Can you work these out from the model? Positions are in its coordinate system, mm. A direction names the side the tool comes from. Round coordinates to 2 decimals unless told otherwise and drop trailing zeros. Loops run counter-clockwise (first coordinate to the right, second up) from the corner with the lowest first, then second, coordinate; pieces in that order, holes last.
(1) Thinking about a two-plate mould opening in Z: for faces 1 (the face through (-44, 4, 2.5)), 2 (the face through (7.27, 2.46, -7.92)), 3 (the face through (-59, 5, 1.7)), 4 (the face through (-61.225, 5, 2)), which applies, released by +Z, released by -Z, zero draft, split by the parting line, or undercut?
(2) I want a section at B-B on x = -23.5. Write out the boundary of the cut face in (y, z).
(3) Which directions (+Z, -Z, +X, -X, +Y, -Y) give clear straight access to the entire face, cutting with the end or side of a thin tool? Please do faces 5 (the face through (-57.604, 4.93, 1.092)), 6 (the face through (-56, 5, 0.5)), 7 (the face through (-61.225, 5, -1)), 8 (the face through (-40.225, 9, 0)), 9 (the face through (-51, 10, -1)).
(4) If I drill on line 1 along X through (y, z) = (3.95, 0); line 2 along Z through (x, y) = (-43, 3.75); line 3 along Z through (x, y) = (-16.5, 3.5), over which ranges is the centre line in solid material (lowest first)?
(5) I want a section at D-D on x = 0. Write out the boundary of the cut face in (y, z).
(6) I want a section at C-C on y = 6. Write out the boundary of the cut face in (x, z), plus the area to 3 significant figures.
(7) Will these pins go through, and if not, where does the flat tip stop? pin 1 Ø12 at (x, z) = (-4.5, 2.5) entering from +Y; pin 2 Ø3 at (x, y) = (-50.5, 5) entering from +Z; pin 3 Ø0.5 at (y, z) = (3.5, 0) entering from -X (3 decimals); pin 4 Ø4 at (y, z) = (5.5, -4) entering from -X (3 decimals).
(8) I want a section at A-A on x = -54. Write out the boundary of the cut face in (y, z).
from build123d import *

# Parameters (mm, degrees)
SKETCH_1_R               = 12
SKETCH_1_R_2             = 10.75
RING_DEPTH               = 5
SKETCH_2_W               = 50
SKETCH_2_H               = 5
STICK_DEPTH              = 5
SKETCH_3_W               = 21
SKETCH_3_H               = 5
KEY_DEPTH                = 10
FILLET_1_R               = 5
FILLET_5_R               = 3
CUT_EXTRUDE_1_DEPTH      = 63.839058045
CUT_EXTRUDE_1_DEPTH_BACK = 63.839058045
FILLET_7_R               = 0.5


with BuildPart() as part:
    # Эскиз1 → ring (new body)
    with BuildSketch(Plane(origin=(0, 0, 0), x_dir=(1, 0, 0), z_dir=(0, 1, 0))):
        with Locations(Location((0, 0, 0), (0, 0, 270))):
            Circle(SKETCH_1_R)
        with Locations(Location((0, 0, 0), (0, 0, 270))):
            Circle(SKETCH_1_R_2, mode=Mode.SUBTRACT)
    extrude(amount=RING_DEPTH)

    # Эскиз2 → stick (add)
    with BuildSketch(Plane(origin=(0, 0, 0), x_dir=(1, 0, 0), z_dir=(0, 1, 0))):
        with Locations((-36.22497216, 0)):
            Rectangle(SKETCH_2_W, SKETCH_2_H)
    extrude(amount=STICK_DEPTH)

    # Эскиз3 → key (add)
    with BuildSketch(Plane(origin=(0, 0, 0), x_dir=(1, 0, 0), z_dir=(0, 1, 0))):
        with Locations((-50.72497216, 0)):
            Rectangle(SKETCH_3_W, SKETCH_3_H)
    extrude(amount=KEY_DEPTH)

    # Скругление1
    fillet_1_edges = [part.edges().sort_by_distance(p)[0] for p in [
        (-11.736694594, 2.5, 2.5),
        (-11.736694594, 2.5, -2.5),
    ]]
    fillet(fillet_1_edges, radius=FILLET_1_R)

    # Скругление5
    fillet_5_edges = [part.edges().sort_by_distance(p)[0] for p in [
        (-40.22497216, 5, 0),
    ]]
    fillet(fillet_5_edges, radius=FILLET_5_R)

    # Эскиз4 → Вытянуть1 (cut, two sides: drawn at the far end of the back side and taken through both)
    with BuildSketch(Plane(origin=(0, 2.5, 0), x_dir=(1, 0, 0), z_dir=(0, 1, 0)).offset(-CUT_EXTRUDE_1_DEPTH_BACK)):
        Polygon((-61.22497216, 0.5), (-41.22497216, 0.5), (-41.22497216, -0.5), (-42.388207879, -0.5), (-42.82497216, -1.7), (-44.62497216, -1.7), (-45.061736441, -0.5), (-46.22497216, -0.5), (-47.388207879, -0.5), (-47.82497216, -1.7), (-49.62497216, -1.7), (-50.061736441, -0.5), (-51.22497216, -0.5), (-52.388207879, -0.5), (-52.82497216, -1.7), (-54.62497216, -1.7), (-55.061736441, -0.5), (-56.22497216, -0.5), (-57.388207879, -0.5), (-57.82497216, -1.7), (-59.62497216, -1.7), (-60.061736441, -0.5), (-61.22497216, -0.5), align=None)
    extrude(amount=CUT_EXTRUDE_1_DEPTH + CUT_EXTRUDE_1_DEPTH_BACK, mode=Mode.SUBTRACT)

    # Скругление7
    fillet_7_edges = [part.edges().sort_by_distance(p)[0] for p in [
        (-38.240559231, 0, 2.5),
        (12, 0, 0),
        (-38.240559231, 0, -2.5),
        (-12.613175603, 0, 3.255626562),
        (-12.613175603, 0, -3.255626562),
    ]]
    fillet(fillet_7_edges, radius=FILLET_7_R)


solid = part.part
Filled sheet:
1. face 1: released by +Z
1. face 2: undercut
1. face 3: undercut
1. face 4: zero draft
2. outline: (0, -2) arc R0.5 ccw to (0.5, -2.5) - (5, -2.5) - (5, 2.5) - (0.5, 2.5) arc R0.5 ccw to (0, 2) - close
3. face 5: +Y, -Y
3. face 6: -X, +Y, -Y
3. face 7: +Z, -Z, -X, +Y, -Y
3. face 8: +Z, -Z, +X, +Y
3. face 9: +Z, -Z, +X, -X, +Y
4. line 1: x = -41.22 to -10.75, 10.75 to 12
4. line 2: z = -2.5 to -0.5, 1.7 to 2.5
4. line 3: z = -2.5 to 2.5
5. outline: (0, -11.5) arc R0.5 ccw to (0.5, -12) - (5, -12) - (5, -10.75) - (0, -10.75) - close; (0, 10.75) - (5, 10.75) - (5, 12) - (0.5, 12) arc R0.5 ccw to (0, 11.5) - close
6. outline: (-61.22, -2.5) - (-39.46, -2.5) - (-39.46, 2.5) - (-61.22, 2.5) - (-61.22, 0.5) - (-60.06, 0.5) - (-59.62, 1.7) - (-57.82, 1.7) - (-57.39, 0.5) - (-55.06, 0.5) - (-54.62, 1.7) - (-52.82, 1.7) - (-52.39, 0.5) - (-50.06, 0.5) - (-49.62, 1.7) - (-47.82, 1.7) - (-47.39, 0.5) - (-45.06, 0.5) - (-44.62, 1.7) - (-42.82, 1.7) - (-42.39, 0.5) - (-41.22, 0.5) - (-41.22, -0.5) - (-61.22, -0.5) - close
6. area: 78.1 mm2
7. pin 1: stops at y = 5
7. pin 2: stops at z = 2.5
7. pin 3: stops at x = -41.225
7. pin 4: stops at x = -61.225
8. outline: (0, -2) arc R0.5 ccw to (0.5, -2.5) - (10, -2.5) - (10, -0.5) - (0, -0.5) - close; (0, 1.7) - (10, 1.7) - (10, 2.5) - (0.5, 2.5) arc R0.5 ccw to (0, 2) - close
